Autodesk Inventor part; units mm, degrees
ref_plane "YZ Plane" through (0, 0, 0) normal (1, 0, 0) x (0, 1, 0)
ref_plane "XZ Plane" through (0, 0, 0) normal (0, 1, 0) x (-1, 0, 0)
ref_plane "XY Plane" through (0, 0, 0) normal (0, 0, 1) x (1, 0, 0)
sketch "スケッチ1" plane through (0, 0, 0) normal (0, 0, 1) x (1, 0, 0)
  line L0 (0, 0) -> (10, 0)
  line L1 (10, 0) -> (10, 17)
  line L2 (10, 17) -> (0, 17)
  line L3 (0, 17) -> (0, 0)
  dimension "d0" = 17
  dimension "d1" = 10
extrude "押し出し1" add sketch "スケッチ1" along normal blind 1.885
sketch "スケッチ2" plane through (0, 0, 1.885) normal (0, 0, 1) x (1, 0, 0)
  line L0 (0, 17) -> (0, 0)
  line L1 (0, 8.5) -> (10, 8.5)
  line L2 (10, 0) -> (10, 17)
  line L3 (10, 17) -> (0, 17)
  line L4 (5, 17) -> (5, 0)
  line L5 (0, 0) -> (10, 0)
  line L6 (0, 17) -> (10, 17)
  point P0 (5, 14.5)
  point P1 (5, 2.5)
  dimension "d4" = 6
hole "穴1" at (5, 14.5, 1.885) at (5, 2.5, 1.885) direction (0, 0, -1) diameter 3.1 end through all
fillet "フィレット1" radius 5 4 edges at (0, 17, 0.9425) (10, 17, 0.9425) (10, 0, 0.9425) (0, 0, 0.9425)
properties part number "link2part4"
Source: CAD feature listing. Evaluate the final solid. Frame: model axes, mm. Coordinates: 2 decimals unless noted, no trailing zeros. Loops run counter-clockwise (first coordinate to the right, second up) from the corner with the lowest first, then second, coordinate; pieces in that order, holes last. Notation, with made-up numbers: (47.25, 70) -> (58.25, 70) arc R28 cw to (58.25, 102) -> close; hole circle Ø4 at (32.5, 12.25). An arc over 180 degrees is marked (long way). Answer in a Markdown table with one row per item. Add a question column.
Q1. Ray query, line 1 along Y through (x, z) = (5, 1.3); line 2 along Y through (x, z) = (3.75, 0.1); line 3 along X through (y, z) = (14.5, 0.5). Return the intervals inside material, ascending.
Q2. Section C-C on x = 5.75. Return the cut outline in (y, z) (1 decimal).
Q3. Pull-direction query (Y, two-part tool) for faces 1 (the face through (5, 9, 1.885)), 2 (the face through (4.93, 16.05, 0.93)), 3 (the face through (9, 15, 1)); classes: pulls with the +Y half, pulls with the -Y half, needs draft (parallel to the pull), parting line crosses it, or undercut.
Q4. Section A-A on z = 1.25. Give the number of separate pieces and of enclosed holes in the cut face, and give its area (3 significant figures).
Q5. Section B-B on y = 2.5. Return the cut outline in (x, z) (3 decimals).
Q6. Section D-D on x = 8.5. Return the cut outline in (y, z) (3 decimals).
Q7. Contact query for a flat-ended pin moving along its axis: pin 1 Ø3 at (x, y) = (5, 14.5) entering from +Z. Output: stop coordinate, or through.
Computed values:
| question | item | result |
|---|---|---|
| 1 | line 1 | y = 0 to 0.95, 4.05 to 12.95, 16.05 to 17 |
| 1 | line 2 | y = 0.16 to 1.58, 3.42 to 13.58, 15.42 to 16.84 |
| 1 | line 3 | x = 0.67 to 3.45, 6.55 to 9.33 |
| 2 | outline | (0.1, 0) -> (1.1, 0) -> (1.1, 1.9) -> (0.1, 1.9) -> close; (3.9, 0) -> (13.1, 0) -> (13.1, 1.9) -> (3.9, 1.9) -> close; (15.9, 0) -> (16.9, 0) -> (16.9, 1.9) -> (15.9, 1.9) -> close |
| 3 | face 1 | needs draft |
| 3 | face 2 | undercut |
| 3 | face 3 | pulls with the +Y half |
| 4 | separate pieces | 1 |
| 4 | enclosed holes | 2 |
| 4 | area | 133 mm^2 |
| 5 | outline | (0.67, 0) -> (3.45, 0) -> (3.45, 1.885) -> (0.67, 1.885) -> close; (6.55, 0) -> (9.33, 0) -> (9.33, 1.885) -> (6.55, 1.885) -> close |
| 6 | outline | (1.429, 0) -> (15.571, 0) -> (15.571, 1.885) -> (1.429, 1.885) -> close |
| 7 | pin 1 | passes through |
